Answer from the drawing. Dimensions are ordinates in mm from the lowest x, y and z of the part. Give positions to 0.01 mm unless a question says otherwise; leave off trailing zeros. Order: outer loops, then holes, each group sorted by start corner. A loop starts at its lowest first (then second) coordinate and runs counter-clockwise, first axis right, second up. Notation, with made-up numbers: (3, -21.5) - (62, -21.5) arc R19 cw to (62, 14.5) - close; hole circle Ø10 at (32, 38). An arc over 180 degrees is marked (long way). Answer in a Markdown table with one row per item. Add a question column.
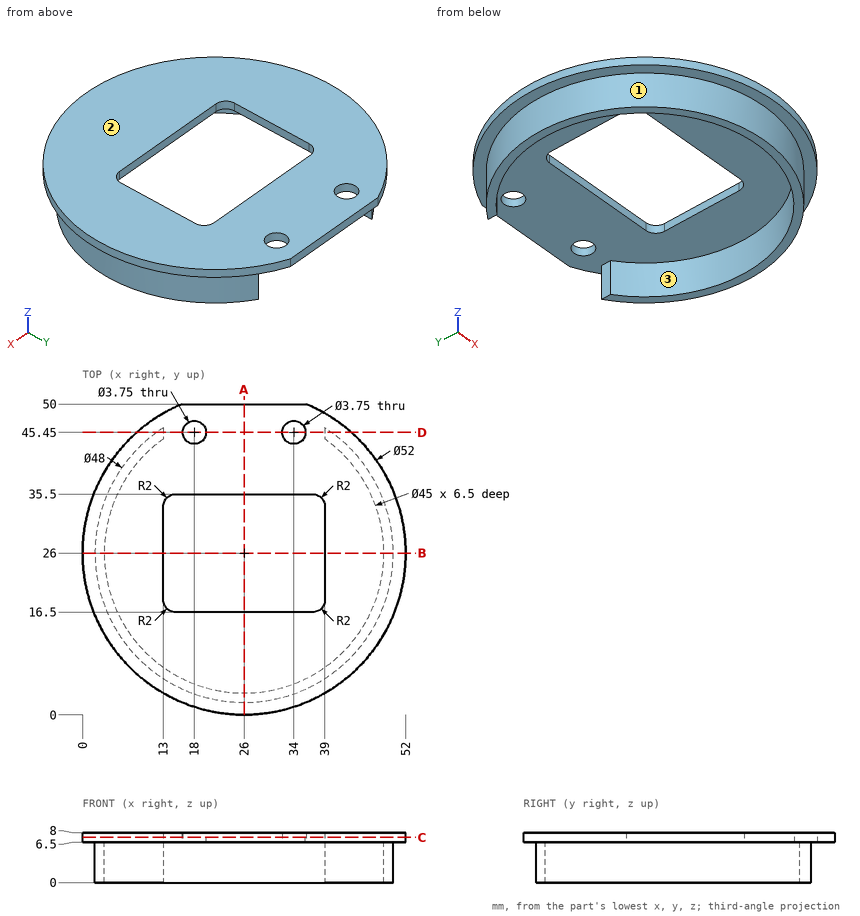
(1) Each of these flat-tipped pins is pushed along its axis until it touches: P1, Ø1.6, axis at y = 28, z = 7.5, coming from the +X side; P2, Ø4, axis at y = 23, z = 6.5, coming from the -X side; P3, Ø0.5, axis at y = 45, z = 3.5, coming from the +X side. Where does it stop, or does it pass through?
(2) Find section B-B, the plane y = 26. Write down the section's boundary in (x, z), plus the area to 3 significant figures.
(3) The mould has two halves that part along X. Classify the marked faces 1, 2 and 3: +X half, -X half, draft (parallel to the pull), parting line (faces both ways), or undercut.
(4) Straight lines are drawn through the part: line 1 (Y direction, x = 34, z = 7.25) (1 decimal); line 2 (Z direction, x = 43.5, y = 17); line 3 (X direction, y = 14, z = 2.5). For each, find the intervals that lie inside material, in ascending order.
(5) Find section C-C, the plane z = 7.25. Write down the section's boundary in (x, y) (3 decimals), plus the area to 3 significant figures.
(6) Find section A-A, the plane x = 26. Write down the section's boundary in (y, z).
(7) Find section D-D, the plane y = 45.45. Write down the section's boundary in (x, z) (1 decimal), plus the area to 3 significant figures.
Answer key:
| question | item | result |
|---|---|---|
| 1 | P1 | x = 51.97 |
| 1 | P2 | x = 0.02 |
| 1 | P3 | x = 40.98 |
| 2 | outline | (0, 6.5) - (2, 6.5) - (2, 0) - (3.5, 0) - (3.5, 6.5) - (13, 6.5) - (13, 8) - (0, 8) - close; (39, 6.5) - (48.5, 6.5) - (48.5, 0) - (50, 0) - (50, 6.5) - (52, 6.5) - (52, 8) - (39, 8) - close |
| 2 | area | 58.5 mm² |
| 3 | face 1 | parting line |
| 3 | face 2 | draft |
| 3 | face 3 | undercut |
| 4 | line 1 | 1.3 to 16.5, 35.5 to 43.6, 47.3 to 50 |
| 4 | line 2 | 6.5 to 8 |
| 4 | line 3 | 5.22 to 6.97, 45.03 to 46.78 |
| 5 | outline | (16, 50) arc R26 ccw (long way) to (36, 50) - close; hole (13, 18.5) arc R2 ccw to (15, 16.5) - (37, 16.5) arc R2 ccw to (39, 18.5) - (39, 33.5) arc R2 ccw to (37, 35.5) - (15, 35.5) arc R2 ccw to (13, 33.5) - close; hole circle Ø3.75 at (18, 45.45); hole circle Ø3.75 at (34, 45.45) |
| 5 | area | 1,580 mm² |
| 6 | outline | (0, 6.5) - (2, 6.5) - (2, 0) - (3.5, 0) - (3.5, 6.5) - (16.5, 6.5) - (16.5, 8) - (0, 8) - close; (35.5, 6.5) - (50, 6.5) - (50, 8) - (35.5, 8) - close |
| 7 | outline | (8.7, 6.5) - (11.9, 6.5) - (11.9, 0) - (13, 0) - (13, 6.5) - (16.1, 6.5) - (16.1, 8) - (8.7, 8) - close; (19.9, 6.5) - (32.1, 6.5) - (32.1, 8) - (19.9, 8) - close; (35.9, 6.5) - (39, 6.5) - (39, 0) - (40.1, 0) - (40.1, 6.5) - (43.3, 6.5) - (43.3, 8) - (35.9, 8) - close |
| 7 | area | 54.3 mm² |
